Input: dimensioned drawing with shaded views. Units: mm. Origin: part minimum x, y, z. A direction names the side the tool comes from. Round coordinates to 2 decimals unless told otherwise and drop trailing zeros. Loops run counter-clockwise (first coordinate to the right, second up) from the corner with the lowest first, then second, coordinate; pieces in that order, holes last. Notation, with made-up numbers: (69.25, -39) - (82.25, -39) arc R20 ccw to (82.25, -18) - close; hole circle Ø8 at (72.25, 19.25). An arc over 180 degrees is marked (long way). Answer as a JSON object with one key per item and string values. Group by question number.
Item 1: Draft query along Y for the marked faces 3, 4, 5 and 6. Return one class per face: released by +Y, released by -Y, zero draft, split by the parting line, or undercut.
Item 2: Section D-D (x = 21). Return the cut outline in (y, z).
Item 3: First-contact query: pin 1 (21 mm diameter, centred on x = 22, z = 25, fed in from -Y); pin 2 (1.6 mm diameter, centred on y = 44, z = 27.5, fed in from -X); pin 3 (3 mm diameter, centred on x = 37.5, z = 37, fed in from +Y). Flat tips, straight axial feed; report the tip coordinate or a pass-through.
Item 4: Line query: line 1 (X direction, y = 1.1, z = 25); line 2 (X direction, y = 1.2, z = 42.5); line 3 (Y direction, x = 55.5, z = 7.5). Output: solid intervals per line, ascending.
Item 5: Section C-C (y = 28.5). Return the cut outline in (x, z).
Item 6: Section A-A (z = 7.5). Return the cut outline in (x, y).
Item 7: Section B-B (x = 39.5). Return the cut outline in (y, z), plus the area to 3 significant figures.
Item 8: Reachability of the marked faces 1 and 2 from +Z, -Z, +X, -X, +Y, -Y: full face, straight path, thin tool, end or side. Return the list, or none.
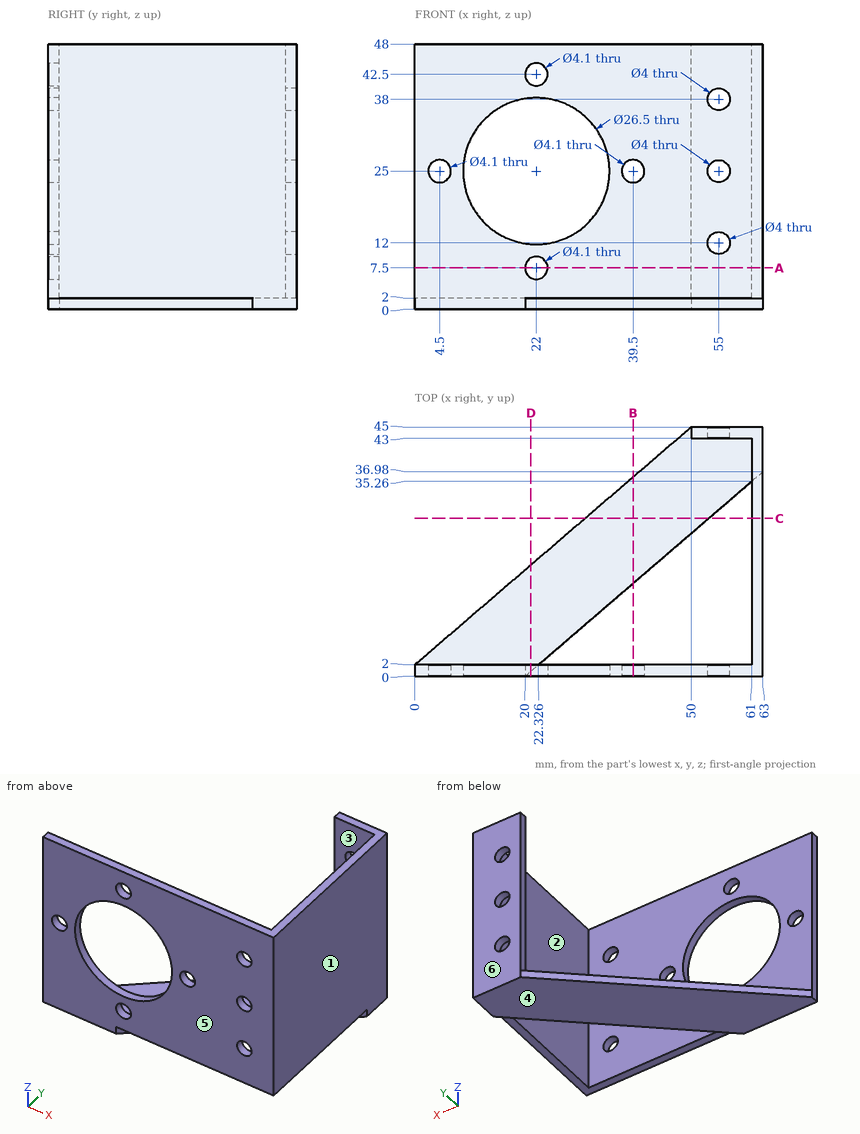
Values:
{
 "1": {"face 3": "undercut", "face 4": "zero draft", "face 5": "released by -Y", "face 6": "released by +Y"},
 "2": {"outline": "(0, 2) - (0.86, 2) - (0.86, 0) - (20.06, 0) - (20.06, 2) - (2, 2) - (2, 5.71) - (0, 5.71) - close; (0, 9.29) - (2, 9.29) - (2, 11.79) - (0, 11.79) - close; (0, 38.21) - (2, 38.21) - (2, 40.71) - (0, 40.71) - close; (0, 44.29) - (2, 44.29) - (2, 48) - (0, 48) - close"},
 "3": {"pin 1": "passes through", "pin 2": "stops at x = 50", "pin 3": "stops at y = 2"},
 "4": {"line 1": "x = 0 to 2.45, 6.55 to 8.75, 35.25 to 37.45, 41.55 to 53, 57 to 63", "line 2": "x = 0 to 19.95, 24.05 to 63", "line 3": "y = 0 to 2, 43 to 45"},
 "5": {"outline": "(30.81, 0) - (53.14, 0) - (53.14, 2) - (30.81, 2) - close; (61, 2) - (63, 2) - (63, 48) - (61, 48) - close"},
 "6": {"outline": "(0, 0) - (19.95, 0) - (19.95, 2) - (0, 2) - close; (24.05, 0) - (63, 0) - (63, 45) - (50, 45) - (50, 43) - (61, 43) - (61, 2) - (24.05, 2) - close"},
 "7": {"outline": "(0, 2) - (2, 2) - (2, 22.95) - (0, 22.95) - close; (0, 27.05) - (2, 27.05) - (2, 48) - (0, 48) - close; (16.77, 0) - (35.97, 0) - (35.97, 2) - (16.77, 2) - close", "area": "122 mm^2"},
 "8": {"face 1": "+Z, -Z, +X, +Y, -Y", "face 2": "+Z, -X"}
}
